Design review of the part built by this model. Coordinates are the model's own, in mm. A direction names the side the tool comes from. Coordinates: 2 decimals unless noted, no trailing zeros. Order: outer loops, then holes, each group sorted by start corner. A loop starts at its lowest first (then second) coordinate and runs counter-clockwise, first axis right, second up. Notation, with made-up numbers: (86.5, 85.5) - (115.5, 85.5) arc R19 cw to (115.5, 115.5) - close; hole circle Ø5 at (50, 2.5). An arc over 180 degrees is marked (long way). Write each question's results on one line, items separated by ' | '. Start each with the question number.
Autodesk Inventor part; units mm, degrees
ref_plane "YZ Plane" through (0, 0, 0) normal (1, 0, 0) x (0, 1, 0)
ref_plane "XZ Plane" through (0, 0, 0) normal (0, 1, 0) x (-1, 0, 0)
ref_plane "XY Plane" through (0, 0, 0) normal (0, 0, 1) x (1, 0, 0)
sketch "Sketch1" plane through (0, 0, 0) normal (0, 1, 0) x (-1, 0, 0)
  line L0 (6.35, -3.6662) -> (0, -7.3323)
  line L1 (0, -7.3323) -> (-6.35, -3.6662)
  line L2 (-6.35, -3.6662) -> (-6.35, 3.6662)
  line L3 (-6.35, 3.6662) -> (0, 7.3323)
  line L4 (0, 7.3323) -> (6.35, 3.6662)
  line L5 (6.35, 3.6662) -> (6.35, -3.6662)
  circle A0 centre (0, 0) radius 38.1
  line L6 (31.5732, -7.3323) -> (25.2232, -3.6662)
  line L7 (25.2232, -3.6662) -> (25.2232, 3.6662)
  line L8 (25.2232, 3.6662) -> (31.5732, 7.3323)
  line L9 (31.5732, 7.3323) -> (37.9232, 3.6662)
  line L10 (37.9232, 3.6662) -> (37.9232, -3.6662)
  line L11 (37.9232, -3.6662) -> (31.5732, -7.3323)
  line L12 (-15.7866, -20.0108) -> (-9.4366, -23.677)
  line L13 (-9.4366, -23.677) -> (-9.4366, -31.0094)
  line L14 (-9.4366, -31.0094) -> (-15.7866, -34.6755)
  line L15 (-15.7866, -34.6755) -> (-22.1366, -31.0094)
  line L16 (-22.1366, -31.0094) -> (-22.1366, -23.677)
  line L17 (-22.1366, -23.677) -> (-15.7866, -20.0108)
  line L18 (-15.7866, 20.0108) -> (-22.1366, 23.677)
  line L19 (-22.1366, 23.677) -> (-22.1366, 31.0094)
  line L20 (-22.1366, 31.0094) -> (-15.7866, 34.6755)
  line L21 (-15.7866, 34.6755) -> (-9.4366, 31.0094)
  line L22 (-9.4366, 31.0094) -> (-9.4366, 23.677)
  line L23 (-9.4366, 23.677) -> (-15.7866, 20.0108)
  circle A1 centre (0, 0) radius 48.26
  circle A2 centre (31.5732, 0) radius 2.9337
  circle A3 centre (-15.7866, -27.3432) radius 2.9337
  circle A4 centre (-15.7866, 27.3432) radius 2.9337
  dimension "d0" = 6.35
  dimension "d1" = 76.2
  dimension "d2" = 120
  dimension "d3" = 120
  dimension "d4" = 10.16
  dimension "d5" = 5.8674
extrude "Extrusion1" add sketch "Sketch1" along normal blind 1.5875 contours A0 L10 | L9 L8 L7 L6 L11 A0 L14 L13 L12 L17 L16 L19 L18 L23 L22 L21 | L10 L11 L6 L7 L8 L9 | L20 A0 | L21 L22 L23 L18 L19 L20 | L15 L16 L17 L12 L13 L14 | A0 L15 | A1
properties part number "spoolEnd"
(1) Take a section at C-C (y = 0.7). State the section outline as (x, z) points, plus the area to 3 significant figures.
(2) Clearance check with a flat-ended pin moving along its axis: pin 1 (7.5 mm diameter, centred on x = 15.79, z = -27.34, fed in from +Y). State where the tip first meets the part, or that it passes through.
(3) Tool access review of faces 4 (the face through (3.219, 0.783, 5.474)), 5 (the face through (1, 1.588, -10)): name each direction out of +Z, -Z, +X, -X, +Y, -Y from which nothing blocks a thin tool from reaching the whole face with its end or side.
(4) Mouldability with a two-part tool opening along Z and no side actions: class faces 1 (the face through (1, 0, -10)), 2 (the face through (-46.03, 0.78, -14.5)), 3 (the face through (3.131, 0.783, -5.525)) as +Z half, -Z half, draft (parallel to the pull), parting line (faces both ways), or undercut.
(5) To check wall thickness, follow line 1 along Z through (x, y) = (17.5, 1.05); line 2 along Z through (x, y) = (17, 0.1); line 3 along X through (y, z) = (0.9, -27). State the ranges of each line that lie inside material, in increasing order. Write a range as [from, to].
(6) Take a section at B-B (x = 14). State the section outline as (y, z) points.
(7) Take a section at D-D (x = 35). State the section outline as (y, z) points, plus the area to 3 significant figures.
(8) Take a section at A-A (z = 0). State the section outline as (x, y) points, plus the area to 3 significant figures.
Worked out:
1) outline: circle Ø96.52 at (0, 0); hole circle Ø5.87 at (-31.57, 0); hole (-6.35, -3.67) - (0, -7.33) - (6.35, -3.67) - (6.35, 3.67) - (0, 7.33) - (-6.35, 3.67) - close; hole circle Ø5.87 at (15.79, -27.34); hole circle Ø5.87 at (15.79, 27.34) | area: 7,100 mm^2
2) pin 1: y = 1.59
3) face 4: +Y, -Y | face 5: +Z, -Z, +X, -X, +Y
4) face 1: draft | face 2: parting line | face 3: undercut
5) line 1: [-44.98, -29.72], [-24.96, 24.96], [29.72, 44.98] | line 2: [-45.17, -30.01], [-24.67, 24.67], [30.01, 45.17] | line 3: [-40, 12.87], [18.7, 40]
6) outline: (0, -46.18) - (1.59, -46.18) - (1.59, -29.67) - (0, -29.67) - close; (0, -25.02) - (1.59, -25.02) - (1.59, 25.02) - (0, 25.02) - close; (0, 29.67) - (1.59, 29.67) - (1.59, 46.18) - (0, 46.18) - close
7) outline: (0, -33.23) - (1.59, -33.23) - (1.59, 33.23) - (0, 33.23) - close | area: 105 mm^2
8) outline: (-48.26, 0) - (-34.51, 0) - (-34.51, 1.59) - (-48.26, 1.59) - close; (-28.64, 0) - (-6.35, 0) - (-6.35, 1.59) - (-28.64, 1.59) - close; (6.35, 0) - (48.26, 0) - (48.26, 1.59) - (6.35, 1.59) - close | area: 124 mm^2
